Read the model definition and answer for the solid it produces. Units are mm, in the model's axes. Coordinates: 2 decimals unless noted, no trailing zeros. Order: outer loops, then holes, each group sorted by start corner. A loop starts at its lowest first (then second) coordinate and runs counter-clockwise, first axis right, second up. Notation, with made-up numbers: (29.5, 14) -> (40.5, 14) arc R28 ccw to (40.5, 49) -> close; hole circle Ø7 at (59.5, 58). An arc over 180 degrees is marked (long way). Return JSON: item names as keys, results as strings. Group by question number.
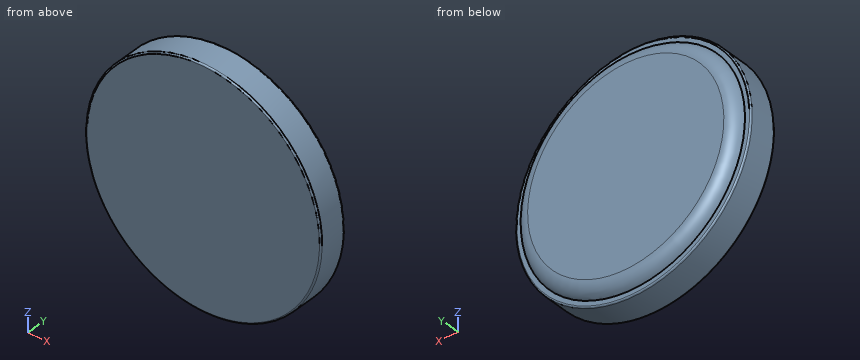
```python
from build123d import *

# Parameters (mm, degrees)
SKETCH1_R           = 10
BOSS_EXTRUDE1_DEPTH = 3.2
CUT_EXTRUDE1_START  = -0.762
SKETCH2_R           = 10
SKETCH2_R_2         = 9.492
CUT_EXTRUDE1_DEPTH  = 0.762
FILLET3_R           = 1.27
FILLET2_R           = 0.127


with BuildPart() as part:
    # Sketch1 → Boss-Extrude1 (new body)
    with BuildSketch(Plane(origin=(0, 0, 0), x_dir=(1, 0, 0), z_dir=(0, 1, 0))):
        with Locations(Location((0, 0, 0), (0, 0, 270))):
            Circle(SKETCH1_R)
    extrude(amount=BOSS_EXTRUDE1_DEPTH)

    # Sketch2 → Cut-Extrude1 (cut)
    with BuildSketch(Plane(origin=(0, 3.2, 0), x_dir=(1, 0, 0), z_dir=(0, 1, 0)).offset(CUT_EXTRUDE1_START)):
        with Locations(Location((0, 0, 0), (0, 0, 270))):
            Circle(SKETCH2_R)
        with Locations(Location((0, 0, 0), (0, 0, 270))):
            Circle(SKETCH2_R_2, mode=Mode.SUBTRACT)
    extrude(amount=CUT_EXTRUDE1_DEPTH, mode=Mode.SUBTRACT)

    # Fillet3
    # the kernel refuses this fillet: 1.27 mm, written as the material it takes off along each edge
    with BuildSketch(Plane(origin=(0, 3.2, 0), x_dir=(0, 0, 1), z_dir=(-1, 0, 0))) as fillet3_piece_1:
        with BuildLine():
            CenterArc((8.328025773, -1.27), FILLET3_R, 23.578178478, 66.421821522)
            Line((8.328025773, 0), (8.328025773, 0.0254))
            Line((8.328025773, 0.0254), (9.492, 0.0254))
            Line((9.492, 0.0254), (9.5174, 0))
            ThreePointArc((9.5174, 0), (9.5174, -0.381), (9.515279485, -0.75184))
            Line((9.515279485, -0.75184), (9.492, -0.762))
        make_face()
    revolve(axis=Axis((0, 3.2, 0), (0, 1, 0)), mode=Mode.SUBTRACT)

    # Fillet2
    fillet2_edges = [part.edges().sort_by_distance(p)[0] for p in [
        (0, 0, -10),
        (0, 2.438, -10),
    ]]
    fillet(fillet2_edges, radius=FILLET2_R)


solid = part.part
```
1. Straight lines are drawn through the part: L1, parallel to X at y = 1.75, z = -0.25; L2, parallel to Z at x = 4, y = 0.7; L3, parallel to X at y = 1.45, z = 8.75. For each, find the intervals that lie inside material, in ascending order.
2. Find section C-C on y = 1.1. Determine the outline of the cut face in (x, z).
3. Find section A-A on x = 0. Determine the outline of the cut face in (y, z).
4. Find section B-B on z = 0. Determine the outline of the cut face in (x, y), and give its area (3 significant figures).
Result:
{
 "1": {"L1": "-10 to 10", "L2": "-9.17 to 9.17", "L3": "-4.84 to 4.84"},
 "2": {"outline": "circle Ø20 at (0, 0)"},
 "3": {"outline": "(0, -9.87) arc R0.13 ccw to (0.13, -10) -> (2.31, -10) arc R0.13 ccw to (2.44, -9.87) -> (2.44, -9.49) arc R1.27 ccw to (3.2, -8.33) -> (3.2, 8.33) arc R1.27 ccw to (2.44, 9.49) -> (2.44, 9.87) arc R0.13 ccw to (2.31, 10) -> (0.13, 10) arc R0.13 ccw to (0, 9.87) -> close"},
 "4": {"outline": "(-10, 0.13) arc R0.13 ccw to (-9.87, 0) -> (9.87, 0) arc R0.13 ccw to (10, 0.13) -> (10, 2.31) arc R0.13 ccw to (9.87, 2.44) -> (9.49, 2.44) arc R1.27 ccw to (8.33, 3.2) -> (-8.33, 3.2) arc R1.27 ccw to (-9.49, 2.44) -> (-9.87, 2.44) arc R0.13 ccw to (-10, 2.31) -> close", "area": "62.7 mm^2"}
}
